```python
from build123d import *

# Parameters (mm, degrees)
SKETCH1_W           = 140
SKETCH1_H           = 55
SKETCH1_R           = 2.65
BOSS_EXTRUDE1_DEPTH = 4
SKETCH2_W           = 140
SKETCH2_H           = 16
BOSS_EXTRUDE2_DEPTH = 10
SKETCH3_W           = 134
SKETCH3_H           = 10
CUT_EXTRUDE1_DEPTH  = 11
CUT_EXTRUDE2_START  = -0.3
SKETCH4_R           = 1.75
CUT_EXTRUDE2_DEPTH  = 76.708223239
FILLET1_R           = 3
FILLET2_R           = 6
FILLET3_R           = 3
CHAMFER1_SIZE       = 1
CHAMFER2_SIZE       = 3


with BuildPart() as part:
    # Sketch1 → Boss-Extrude1 (new body)
    with BuildSketch(Plane.XY):
        Rectangle(SKETCH1_W, SKETCH1_H)
        with Locations((-60, 21.5)):
            Circle(SKETCH1_R, mode=Mode.SUBTRACT)
        with Locations((60, 21.5)):
            Circle(SKETCH1_R, mode=Mode.SUBTRACT)
    extrude(amount=BOSS_EXTRUDE1_DEPTH)

    # Sketch2 → Boss-Extrude2 (add)
    with BuildSketch(Plane.XY.offset(4)):
        with Locations((0, -19.5)):
            Rectangle(SKETCH2_W, SKETCH2_H)
    extrude(amount=BOSS_EXTRUDE2_DEPTH)

    # Sketch3 → Cut-Extrude1 (cut)
    with BuildSketch(Plane(origin=(0, 0, 0), x_dir=(-1, 0, 0), z_dir=(0, 0, -1))):
        with Locations((0, -19.5)):
            Rectangle(SKETCH3_W, SKETCH3_H)
    extrude(amount=-CUT_EXTRUDE1_DEPTH, mode=Mode.SUBTRACT)

    # Sketch4 → Cut-Extrude2 (cut, through all)
    with BuildSketch(Plane(origin=(0, 0, 11), x_dir=(-1, 0, 0), z_dir=(0, 0, -1)).offset(CUT_EXTRUDE2_START)):
        with Locations((52.5, -19.5)):
            Circle(SKETCH4_R)
        with Locations((-52.5, -19.5)):
            Circle(SKETCH4_R)
    extrude(amount=-CUT_EXTRUDE2_DEPTH, mode=Mode.SUBTRACT)

    # Fillet1
    fillet1_edges = [part.edges().sort_by_distance(p)[0] for p in [
        (67, -14.5, 5.5),
        (67, -24.5, 5.5),
        (-67, -24.5, 5.5),
        (-67, -14.5, 5.5),
    ]]
    fillet(fillet1_edges, radius=FILLET1_R)

    # Fillet2
    fillet2_edges = [part.edges().sort_by_distance(p)[0] for p in [
        (70, -11.5, 9),
        (-70, -11.5, 9),
        (70, -27.5, 7),
        (-70, -27.5, 7),
        (-70, 27.5, 2),
        (70, 27.5, 2),
    ]]
    fillet(fillet2_edges, radius=FILLET2_R)

    # Fillet3
    fillet3_edges = [part.edges().sort_by_distance(p)[0] for p in [
        (68.242640687, -13.257359313, 4),
        (0, -11.5, 4),
        (-68.242640687, -13.257359313, 4),
    ]]
    fillet(fillet3_edges, radius=FILLET3_R)

    # Chamfer1
    chamfer1_edges = [part.edges().sort_by_distance(p)[0] for p in [
        (0, -14.5, 11),
        (-67, -19.5, 11),
        (67, -19.5, 11),
        (0, -24.5, 11),
        (66.121320344, -15.378679656, 11),
        (66.121320344, -23.621320344, 11),
        (-66.121320344, -23.621320344, 11),
        (-66.121320344, -15.378679656, 11),
    ]]
    chamfer(chamfer1_edges, length=CHAMFER1_SIZE)

    # Chamfer2
    chamfer2_edges = [part.edges().sort_by_distance(p)[0] for p in [
        (-70, -19.5, 14),
        (0, -11.5, 14),
        (70, -19.5, 14),
        (0, -27.5, 14),
        (68.242640687, -25.742640687, 14),
        (68.242640687, -13.257359313, 14),
        (-68.242640687, -25.742640687, 14),
        (-68.242640687, -13.257359313, 14),
    ]]
    chamfer(chamfer2_edges, length=CHAMFER2_SIZE)


solid = part.part
```
CAD build for the part. Positions are in the model's coordinates, mm. A direction names the side the tool comes from. Coordinates: 2 decimals unless noted, no trailing zeros. Order: outer loops, then holes, each group sorted by start corner. A loop starts at its lowest first (then second) coordinate and runs counter-clockwise, first axis right, second up.
(1) Which spindle directions (+Z, -Z, +X, -X, +Y, -Y) get a long thin tool onto all of the face, cutting with end or side? Do faces 1 (the face through (-68.289, -13.304, 9.028)), 2 (the face through (53, -19, 11.3)), 3 (the face through (70, -5, 3)), 4 (the face through (1, -14.5, 5)), 5 (the face through (-1, -27.5, 5)). Say none if no direction does.
Solution:
face 1: +Z, -X, +Y
face 2: +Z
face 3: +Z, -Z, +X, +Y, -Y
face 4: -Z
face 5: +Z, -Z, +X, -X, -Y
(2) Saw through at D-D, the plane y = 9. Write the cut outline in (x, z), and give its area (3 significant figures).
Solution:
outline: (-70, 0) - (70, 0) - (70, 4) - (-70, 4) - close
area: 560 mm2
(3) Pin check, flat tips, straight feed: pin 1 Ø1.2 at (x, z) = (21, 8) entering from +Y; pin 2 Ø2 at (x, y) = (-52.5, -19.5) entering from +Z; pin 3 Ø2.5 at (x, y) = (-2, -20.5) entering from -Z; pin 4 Ø3 at (x, y) = (-60, 21.5) entering from -Z. Stop position of each tip, or through.
Solution:
pin 1: stops at y = -11.5
pin 2: stops at z = 11.3
pin 3: stops at z = 11
pin 4: passes through
(4) Mould opens along X. For faces 6 (the face through (-1, -19, 14)), 7 (the face through (-66.14, -23.6, 5.07)), 8 (the face through (66.899, -14.537, 12.854)) say: released by +X, released by -X, zero draft, split by the parting line, or undercut.
Solution:
face 6: zero draft
face 7: undercut
face 8: released by +X
(5) Saw through at A-A, the plane x = -60. Write the cut outline in (y, z), and give its area (3 significant figures).
Solution:
outline: (-27.5, 0) - (-24.5, 0) - (-24.5, 10) - (-23.5, 11) - (-15.5, 11) - (-14.5, 10) - (-14.5, 0) - (18.85, 0) - (18.85, 4) - (-8.5, 4) arc R3 cw to (-11.5, 7) - (-11.5, 11) - (-14.5, 14) - (-24.5, 14) - (-27.5, 11) - close; (24.15, 0) - (27.5, 0) - (27.5, 4) - (24.15, 4) - close
area: 243 mm2
(6) Saw through at C-C, the plane y = -19.5. Write the cut outline in (x, z).
Solution:
outline: (-70, 0) - (-67, 0) - (-67, 10) - (-66, 11) - (66, 11) - (67, 10) - (67, 0) - (70, 0) - (70, 11) - (67, 14) - (54.25, 14) - (54.25, 11.3) - (50.75, 11.3) - (50.75, 14) - (-50.75, 14) - (-50.75, 11.3) - (-54.25, 11.3) - (-54.25, 14) - (-67, 14) - (-70, 11) - close
(7) Saw through at B-B, the plane x = 56. Write the cut outline in (y, z).
Solution:
outline: (-27.5, 0) - (-24.5, 0) - (-24.5, 10) - (-23.5, 11) - (-15.5, 11) - (-14.5, 10) - (-14.5, 0) - (27.5, 0) - (27.5, 4) - (-8.5, 4) arc R3 cw to (-11.5, 7) - (-11.5, 11) - (-14.5, 14) - (-24.5, 14) - (-27.5, 11) - close
(8) Drill centre lines: L1, parallel to Y at x = 34.5, z = 2.75; L2, parallel to Y at x = 23, z = 9; L3, parallel to Z at x = -10, y = 23. Where is each one in solid material? Low to high.
Solution:
L1: y = -27.5 to -24.5, -14.5 to 27.5
L2: y = -27.5 to -24.5, -14.5 to -11.5
L3: z = 0 to 4
